Here's how the part is built. I have some questions about the finished solid (model axes, mm). A direction names the side the tool comes from. Coordinates: 2 decimals unless noted, no trailing zeros. Write each loop counter-clockwise with the first axis right and the second up, starting at its lowest first coordinate (ties: lowest second). Pieces come first, ordered by that corner, then holes. Notation, with made-up numbers: (-34.5, -14) - (-16.5, -14) arc R18 ccw to (-16.5, -2) - close; hole circle Ø1 at (63.5, -11.75). An arc over 180 degrees is marked (long way). Answer in a Markdown table with one row per item. Add a question column.
Item 1: Which directions (+Z, -Z, +X, -X, +Y, -Y) give clear straight access to the entire face, cutting with the end or side of a thin tool? Please do faces 1 (the face through (-43, 29.76, -10)), 2 (the face through (-43, 27.76, -10)), 3 (the face through (3, 27.76, -10)).
Item 2: We'd pull the mould along Z, two halves only. Please class faces 4 (the face through (7.275, 29, -18)), 5 (the face through (2.17, 28.75, -4.9)), 6 (the face through (-12.11, 44.05, -7.99)), 7 (the face through (2.17, 28.75, -14.9)): +Z half, -Z half, draft (parallel to the pull), parting line (faces both ways), or undercut.
Item 3: Imagine slicing it at A-A (z = -1.25). Please give me the cut outline in (x, y) (3 decimals), plus the area to 3 significant figures.
Item 4: If I drill on probe 1 along Y at (x, z) = (4.5, -18.75); probe 2 along Y at (x, z) = (-0.5, -10.5); probe 3 along X at (y, z) = (4, -5.75), over which ranges is the centre line in solid material (lowest first)? Write a range as from..to.
Item 5: Imagine slicing it at C-C (y = 29). Please give me the cut outline in (x, z) (3 decimals), plus the area to 4 significant figures.
Item 6: Imagine slicing it at D-D (z = -15.02). Please give me the cut outline in (x, y).
Item 7: I'm going to push flat-ended pins straight in: pin 1 (6 mm diameter, centred on y = 17.5, z = -5.5, fed in from +X); pin 2 (8.5 mm diameter, centred on x = -44.63, z = -5.02, fed in from -Y); pin 3 (1.6 mm diameter, centred on x = 2.5, y = 28.5, fed in from -Z). Where does each tip first touch, or does it pass through?
Item 8: Imagine slicing it at B-B (x = -9.9). Please give me the cut outline in (y, z), plus the area to 3 significant figures.
Autodesk Inventor part; units mm, degrees
ref_plane "YZ Plane" through (0, 0, 0) normal (1, 0, 0) x (0, 1, 0)
ref_plane "XZ Plane" through (0, 0, 0) normal (0, 1, 0) x (-1, 0, 0)
ref_plane "XY Plane" through (0, 0, 0) normal (0, 0, 1) x (1, 0, 0)
sketch "スケッチ1" plane through (0, 0, 0) normal (0, 1, 0) x (-1, 0, 0)
  line L0 (0, 0) -> (39.83, 0)
  line L1 (39.83, 0) -> (39.83, -20.04)
  line L2 (39.83, -20.04) -> (0, -20.04)
  line L3 (0, -20.04) -> (0, 0)
  dimension "d0" = 39.83
  dimension "d1" = 20.04
extrude "押し出し1" add sketch "スケッチ1" along normal blind 40.4
ref_plane "作業平面2" through (0, 27.76, 0) normal (0, -1, 0) x (1, 0, 0)
sketch "スケッチ3" plane through (0, 27.76, 0) normal (0, -1, 0) x (1, 0, 0)
  line L0 (0, 0) -> (7.275, 0)
  line L1 (7.275, 0) -> (7.275, -20.0108)
  line L2 (7.275, -20.0108) -> (0, -20.0108)
  line L3 (0, -20.0108) -> (0, 0)
  line L4 (-39.83, -20.04) -> (-39.83, 0)
  line L5 (-39.83, 0) -> (-47.105, 0)
  line L6 (-47.105, 0) -> (-47.105, -20.04)
  line L7 (-47.105, -20.04) -> (-39.83, -20.04)
  line L8 (-39.83, -20.04) -> (-39.83, 0)
  dimension "d5" = 7.275
  dimension "d6" = 20.0108
  dimension "d7" = 7.275
extrude "押し出し2" add sketch "スケッチ3" against normal blind 2
sketch "スケッチ6" plane through (0, 40.4, 0) normal (0, 1, 0) x (1, 0, 0)
  line L0 (0, 0) -> (0, 20.04)
  line L1 (0, 0) -> (0, 20.04)
  line L2 (-39.83, 20.04) -> (-39.83, 0)
  line L3 (-39.83, 10.02) -> (0, 10.02)
  circle A0 centre (-9.9, 10.02) radius 3
  dimension "d11" = 9.9
  dimension "d12" = 6
extrude "押し出し3" add sketch "スケッチ6" along normal blind 7.4
sketch "スケッチ9" plane through (0, 29.76, 0) normal (0, 1, 0) x (1, 0, 0)
  circle A0 centre (-44.6339, 15.02) radius 2.75
  circle A1 centre (-44.6339, 5.02) radius 2.75
  circle A2 centre (4.8661, 15.0054) radius 2.75
  circle A3 centre (4.8661, 5.0054) radius 2.75
  line L0 (-47.105, 0) -> (-47.105, 20.04)
  line L1 (-47.105, 10.02) -> (-39.83, 10.02)
  line L2 (-39.83, 20.04) -> (-39.83, 0)
  line L3 (-47.105, 20.04) -> (-47.105, 0)
  line L4 (-44.6339, 15.02) -> (-44.6339, 5.02)
  line L5 (4.8661, 15.0054) -> (4.8661, 5.0054)
  line L6 (7.275, 20.0108) -> (7.275, 0)
  line L7 (7.275, 10.0054) -> (0.184, 10.0054)
  point P0 (0, 0)
  point P1 (-44.6339, 10.02)
  point P2 (4.8661, 10.0054)
  dimension "d15" = 10
  dimension "d16" = 5.5
  dimension "d17" = 5.5
  dimension "d18" = 5.5
  dimension "d19" = 10
  dimension "d20" = 5.5
  dimension "d21" = 49.5
hole "穴1" at (-44.6339, 29.76, -15.02) at (4.8661, 29.76, -15.0054) at (-44.6339, 29.76, -5.02) at (4.8661, 29.76, -5.0054) direction (0, -1, 0) diameter 5.4 end through all
properties part number "sarvo_motor"
Here are the results:
| question | item | result |
|---|---|---|
| 1 | face 1 | +Z, -Z, -X, +Y |
| 1 | face 2 | +Z, -Z, -X, -Y |
| 1 | face 3 | +Z, -Z, +X, -Y |
| 2 | face 4 | draft |
| 2 | face 5 | undercut |
| 2 | face 6 | parting line |
| 2 | face 7 | undercut |
| 3 | outline | (-47.105, 27.76) - (-39.83, 27.76) - (-39.83, 0) - (0, 0) - (0, 27.76) - (7.275, 27.76) - (7.275, 29.76) - (0, 29.76) - (0, 40.4) - (-39.83, 40.4) - (-39.83, 29.76) - (-47.105, 29.76) - close |
| 3 | area | 1,640 mm2 |
| 4 | probe 1 | y = 27.76..29.76 |
| 4 | probe 2 | y = 0..40.4 |
| 4 | probe 3 | x = -39.83..0 |
| 5 | outline | (-47.105, -20.04) - (0, -20.04) - (0, -20.011) - (7.275, -20.011) - (7.275, -16.225) arc R2.7 cw (long way) to (7.275, -13.786) - (7.275, -6.225) arc R2.7 cw (long way) to (7.275, -3.786) - (7.275, 0) - (-47.105, 0) - (-47.105, -3.932) arc R2.7 cw (long way) to (-47.105, -6.108) - (-47.105, -13.932) arc R2.7 cw (long way) to (-47.105, -16.108) - close |
| 5 | area | 1,000 mm2 |
| 6 | outline | (-41.93, 27.76) - (-39.83, 27.76) - (-39.83, 0) - (0, 0) - (0, 27.76) - (2.17, 27.76) - (2.17, 29.76) - (0, 29.76) - (0, 40.4) - (-39.83, 40.4) - (-39.83, 29.76) - (-41.93, 29.76) - close |
| 7 | pin 1 | stops at x = 0 |
| 7 | pin 2 | stops at y = 27.76 |
| 7 | pin 3 | stops at z = -20.01 |
| 8 | outline | (0, -20.04) - (40.4, -20.04) - (40.4, -13.02) - (47.8, -13.02) - (47.8, -7.02) - (40.4, -7.02) - (40.4, 0) - (0, 0) - close |
| 8 | area | 854 mm2 |
